Autodesk Inventor part; units mm, degrees
ref_plane "YZ Plane" through (0, 0, 0) normal (1, 0, 0) x (0, 1, 0)
ref_plane "XZ Plane" through (0, 0, 0) normal (0, 1, 0) x (-1, 0, 0)
ref_plane "XY Plane" through (0, 0, 0) normal (0, 0, 1) x (1, 0, 0)
sketch "Skizze1" plane through (0, 0, 0) normal (0, 0, 1) x (1, 0, 0)
  line L0 (-17, 0) -> (-25, 0)
  line L1 (-25, 0) -> (-25, -23)
  line L2 (-23, -25) -> (0, -25)
  line L3 (0, -25) -> (0, -17)
  line L4 (-17, 0) -> (-17, -15)
  line L5 (-15, -17) -> (0, -17)
  arc A0 (-25, -23) -> (-23, -25) centre (-23, -23) ccw construction
  circle A1 centre (-20.8, -14.5) radius 2.4
  circle A2 centre (-14.5, -20.8) radius 2.4
  arc A3 (-17, -15) -> (-15, -17) centre (-15, -15) ccw
  circle A4 centre (-14.5, -20.8) radius 2.4 construction
  circle A5 centre (-20.8, -14.5) radius 2.4 construction
  line L6 (-30.4971, 0) -> (5.0828, 0) construction
  line L7 (0, -30.4971) -> (0, 5.0828) construction
  line L8 (-23, -25) -> (-25, -25)
  line L9 (-25, -23) -> (-25, -25)
  line L10 (0, -17) -> (0, 0)
  line L11 (0, 0) -> (-17, 0)
  point P0 (-17, -17)
  dimension "d278" = 25
  dimension "d279" = 25
  dimension "d2" = 8
  dimension "d281" = 8
  dimension "d282" = 2
  dimension "d286" = 4.8
  dimension "d_hole" = 4.8
  dimension "d290" = 20.8
  dimension "d" = 20.8
  dimension "d292" = 2
  dimension "d313" = 6.3
  dimension "d314" = 6.3
  dimension "d332" = 0
extrude "Extrusion1" add sketch "Skizze1" along normal blind 5
mirror "Mirror6" about plane through (0, 0, 0) normal (0, 1, 0) of "Extrusion1"
sketch "Sketch26" plane through (0, 0, 5) normal (0, 0, 1) x (1, 0, 0)
  line L0 (-25, 25) -> (0, 25)
  line L1 (-25, -25) -> (-25, 25)
  line L2 (-25, -25) -> (0, -25)
  line L3 (-25, -23) -> (-25, 23)
  line L4 (-28.6, -7) -> (-28.6, -7)
  line L5 (-30.6, -5) -> (-30.6, 5)
  line L6 (-28.6, 7) -> (-28.6, 7)
  line L7 (-25, 16.8311) -> (-25, -7)
  line L8 (-26.3639, 5) -> (-25, 5)
  line L9 (-25, -5) -> (-26.3639, -5)
  arc A0 (-30.6, -5) -> (-28.6, -7) centre (-28.6, -5) ccw
  arc A1 (-28.6, -7) -> (-26.6124, -5.2222) centre (-28.6, -5) ccw
  arc A2 (-28.6, 7) -> (-30.6, 5) centre (-28.6, 5) ccw
  arc A3 (-26.6124, 5.2222) -> (-28.6, 7) centre (-28.6, 5) ccw
  arc A4 (-26.3639, -5) -> (-26.6124, -5.2222) centre (-26.3639, -5.25) ccw
  arc A5 (-26.6124, 5.2222) -> (-26.3639, 5) centre (-26.3639, 5.25) ccw
  line L10 (-37.2171, 0) -> (6.2028, 0)
  line L11 (0, -25) -> (0, 25)
  point P0 (0, 0)
  point P1 (-24.0313, 1.861)
  point P2 (-28.6, -7)
  point P3 (-25, -5)
  point P4 (-25, 5)
  point P5 (-28.6, 7)
  dimension "d293" = 5.6
  dimension "d300" = 2
  dimension "d301" = 0.25
  dimension "d365" = 7
  dimension "d367" = 7
  dimension "d385" = 5
  dimension "d386" = 5
extrude "Extrusion13" add sketch "Sketch26" against normal up to surface (5 mm away) contours L10 L5 A2 A3 A5 L8 L1 | L1 L9 A4 A1 A0 L5 L10
sketch "Skizze36" plane through (0, 0, 5) normal (0, 0, 1) x (1, 0, 0)
  line L0 (30.9789, 27.5712) -> (-10, 27.5712)
  line L1 (-10, 27.5712) -> (-10, -32.2955)
  line L2 (-10, -32.2955) -> (30.9789, -32.2955)
  line L3 (30.9789, -32.2955) -> (30.9789, 27.5712)
  line L4 (-25, 23) -> (-25, 5)
  point P0 (0, 0)
  dimension "d401" = 15
extrude "Extrusion19" cut sketch "Skizze36" against normal blind 10
pattern_linear "Rechteckige Anordnung8" count 3 spacing 50 along (0, 1, 0) of "Extrusion1", "Mirror6", "Extrusion13", "Extrusion19"
fillet "Rundung6" radius 2 2 edges at (-25, -25, 2.5) (-25, 125, 2.5)
sketch "Skizze37" plane through (0, 0, 0) normal (0, 0, -1) x (-1, 0, 0)
  arc A0 (23.1, -20.49) -> (20.5755, -23.0145) centre (21.2, -21.1145) ccw
  arc A1 (20.7515, 22.8345) -> (23.1, 20.261) centre (21.2, 20.8855) ccw
  arc A2 (23.1, 29.51) -> (20.5755, 26.9855) centre (21.2, 28.8855) ccw
  arc A3 (20.7515, 72.8345) -> (23.1, 70.261) centre (21.2, 70.8855) ccw
  arc A4 (23.1, 79.51) -> (20.5755, 76.9855) centre (21.2, 78.8855) ccw
  arc A5 (20.7515, 122.8345) -> (23.1, 120.261) centre (21.2, 120.8855) ccw
  point P0 (0, 0)
hole "Bohrung8" at (-21.2, 120.8855, 0) at (-21.2, 78.8855, 0) at (-21.2, 70.8855, 0) at (-21.2, 28.8855, 0) at (-21.2, 20.8855, 0) at (-21.2, -21.1145, 0) direction (0, 0, 1) diameter 3.2 end through all
equation "\"d_i\" = 40"
equation "\"d_o\" = 40"
equation "\"d_part\" = 50"
equation "\"d6\" = 0"
equation "\"d7\" = 0"
equation "\"d8\" = 0"
equation "\"d9\" = 0"
equation "\"d13\" = 0"
equation "\"d14\" = 0"
equation "\"d20\" = 0"
equation "\"d21\" = 0"
equation "\"d22\" = 0"
equation "\"d23\" = 0"
equation "\"d24\" = 0"
equation "\"d25\" = 3"
equation "\"d26\" = 0"
equation "\"d27\" = 0"
equation "\"d28\" = 0"
equation "\"d29\" = 0"
equation "\"d30\" = 0"
equation "\"d31\" = 0"
equation "\"d32\" = 0"
equation "\"d33\" = 0"
equation "\"d34\" = 0"
equation "\"d46\" = 0"
equation "\"d47\" = 0"
equation "\"d48\" = 0"
equation "\"d50\" = 0"
equation "\"d51\" = 0"
equation "\"d52\" = 0"
equation "\"d53\" = 0"
equation "\"d54\" = 0"
equation "\"d55\" = 0"
equation "\"d56\" = 0"
equation "\"d57\" = 0"
equation "\"d58\" = 0"
equation "\"d59\" = 0"
equation "\"magnet_offset\" = 0"
equation "\"screw_offset\" = 0"
equation "\"mal_puzzle_offset\" = 0"
equation "\"fem_puzzle_offset\" = 0"
properties part number "40_Cube_XY_Table_Aliexpress_naked_puzzlebar"
Design review of the part built by this model. Coordinates are the model's own, in mm. Give positions to 0.01 mm unless a question says otherwise; leave off trailing zeros. Order: outer loops, then holes, each group sorted by start corner. A loop starts at its lowest first (then second) coordinate and runs counter-clockwise, first axis right, second up. Notation, with made-up numbers: (78.5, 3.5) - (114.5, 3.5) arc R13 cw to (114.5, 14.5) - close; hole circle Ø4 at (87, 84.5). An arc over 180 degrees is marked (long way). Write item = value, one per line. Start each with the question number.
Q1. Clearance check with flat-ended pins moving along their axes: pin 1 Ø1.5 at (y, z) = (92.5, 3) entering from -X; pin 2 Ø1.5 at (x, z) = (-25.5, 2.5) entering from -Y; pin 3 Ø1.5 at (x, z) = (-25.5, 1.5) entering from +Y. State where each tip first meets the part, or that it passes through.
Q2. We need section C-C on z = 2.7. State how many separate pieces and enclosed holes the cut face has, plus the area to 3 significant figures.
Q3. Mouldability with a two-part tool opening along X and no side actions: class faces 1 (the face through (-10, 51, 3)), 2 (the face through (-21.11, 112.12, 2.46)), 3 (the face through (-30.6, 50, 3)), 4 (the face through (-15.02, 123.143, 2.465)) as released by +X, released by -X, zero draft, split by the parting line, or undercut.
Q4. To check wall thickness, follow L1, parallel to X at y = 20.8, z = 3.2; L2, parallel to X at y = 27.5, z = 2.15; L3, parallel to Y at x = -26.5, z = 4.05. State the ranges of each line that lie inside material, in increasing order. Write a range as from..to.
Q5. We need section A-A on y = 85.5. State the section outline as (x, z) points.
Q6. We need section B-B on y = -20.8. State the section outline as (x, z) points.
Working result:
q1.pin_1 = -29.57
q1.pin_2 = -23.97
q1.pin_3 = 123.97
q2.separate_pieces = 1
q2.enclosed_holes = 18
q2.area = 2,190 mm²
q3.face_1 = released by +X
q3.face_2 = undercut
q3.face_3 = released by -X
q3.face_4 = undercut
q4.L1 = -25..-22.8, -19.6..-16.9, -12.1..-10
q4.L2 = -25..-22, -20.4..-16.19, -12.81..-10
q4.L3 = -5.04..5.04, 44.96..55.04, 94.96..105.04
q5.outline = (-25, 0) - (-23.2, 0) - (-23.2, 5) - (-25, 5) - close; (-18.4, 0) - (-10, 0) - (-10, 5) - (-18.4, 5) - close
q6.outline = (-25, 0) - (-22.77, 0) - (-22.77, 5) - (-25, 5) - close; (-19.63, 0) - (-16.9, 0) - (-16.9, 5) - (-19.63, 5) - close; (-12.1, 0) - (-10, 0) - (-10, 5) - (-12.1, 5) - close
